Could you check a few things on this model? Use its own coordinates, in mm. A direction names the side the tool comes from. Give positions to 0.01 mm unless a question says otherwise; leave off trailing zeros. Loops run counter-clockwise (first coordinate to the right, second up) from the corner with the lowest first, then second, coordinate; pieces in that order, holes last. Notation, with made-up numbers: (-27.5, 33.25) - (-17.5, 33.25) arc R25 cw to (-17.5, 47.25) - close; hole circle Ø7 at (-14, 12). An arc over 180 degrees is marked (long way). Use CSV: the item, a comma, the result in double quotes.
from build123d import *

# Parameters (mm, degrees)
F0_W     = 127
F0_H     = 127
F1_DEPTH = 127
F2_R     = 32.47457
F3_DEPTH = 93.218


with BuildPart() as f1:
    # F0 (on Top) → F1 (new body)
    with BuildSketch(Plane.XY):
        with Locations((0, -63.5)):
            Rectangle(F0_W, F0_H)
    extrude(amount=F1_DEPTH)

    # F2 (on face) → F3 (join)
    with BuildSketch(Plane.YZ.offset(63.5)):
        with Locations((-63.9963, 58.810309)):
            Circle(F2_R)
    extrude(amount=F3_DEPTH)


solid = f1.part
1) Suppose I cut it at A-A (z = 89). Please give me the cut outline in (x, y), plus the area to 3 significant figures.
Answer below:
outline,"(-63.5, -127) - (63.5, -127) - (63.5, -75.96) - (156.72, -75.96) - (156.72, -52.03) - (63.5, -52.03) - (63.5, 0) - (-63.5, 0) - close"
area,"18,400 mm2"
2) Suppose I cut it at D-D (y = -118.5). Please give me the cut outline in (x, z).
Answer below:
outline,"(-63.5, 0) - (63.5, 0) - (63.5, 127) - (-63.5, 127) - close"
3) Suppose I cut it at C-C (x = 117.5). Please give me the cut outline in (y, z), plus the area to 3 significant figures.
Answer below:
outline,"circle Ø64.95 at (-64, 58.81)"
area,"3,310 mm2"
4) I need wall thicknesses on line 1 along X through (y, z) = (-13.5, 9.5); line 2 along Z through (x, y) = (114, -74); line 3 along Y through (x, z) = (148, 75). Which ranges of each line are inside material? Lowest first, please.
Answer below:
line 1,"x = -63.5 to 63.5"
line 2,"z = 27.91 to 89.71"
line 3,"y = -92.15 to -35.85"
5) Which directions (+Z, -Z, +X, -X, +Y, -Y) give clear straight access to the entire face, cutting with the end or side of a thin tool? Please do faces 1 (the flat face through (-1, -63, 0)), 2 (the flat face through (63.5, -79, 91)).
Answer below:
face 1,"-Z, +X, -X, +Y, -Y"
face 2,"+X"
6) Suppose I cut it at B-B (y = -57). Please give me the cut outline in (x, z).
Answer below:
outline,"(-63.5, 0) - (63.5, 0) - (63.5, 27.1) - (156.72, 27.1) - (156.72, 90.52) - (63.5, 90.52) - (63.5, 127) - (-63.5, 127) - close"
